from build123d import *
from OCP.BRepFilletAPI import BRepFilletAPI_MakeChamfer

# Parameters (mm, degrees)
BOSS_EXTRUDE1_DEPTH       = 33.86758938
F_1_4_CLEARANCE_HOLE1_D   = 7.14248
DRAFT1_ANGLE              = 15
DRAFT2_ANGLE              = 15
DRAFT3_ANGLE              = 5
DRAFT4_ANGLE              = 5
CHAMFER1_SIZE             = 2.54
CHAMFER1_SIZE2            = 2.599295174
CHAMFER2_SIZE             = 1.27
CHAMFER2_SIZE2            = 1.356155551
CHAMFER2_SIZE2_2          = 1.397079842
CHAMFER2_SIZE2_3          = 1.796051224
CHAMFER2_SIZE2_4          = 1.739452222
HOLE1_AT_2_COUNT          = 2
HOLE1_AT_2_PITCH          = 24.154432116
F_8_CLEARANCE_HOLE1_D     = 4.9149
F_8_CLEARANCE_HOLE1_DEPTH = 9.525
F_8_CLEARANCE_HOLE1_TIP   = 1.476584928


with BuildPart() as part:
    # Sketch1 → Boss-Extrude1 (new body)
    with BuildSketch(Plane.XY):
        Polygon((133.529465969, -12.7), (114.479465969, -12.7), (114.479465969, -8.89), (111.939465969, -6.35), (107.494465969, -6.35), (104.954465969, -6.35), (104.954465969, -25.4), (143.054465969, -25.4), (143.054465969, -6.35), (140.514465969, -6.35), (136.069465969, -6.35), (133.529465969, -8.89), align=None)
    extrude(amount=-BOSS_EXTRUDE1_DEPTH)

    # 1/4 Clearance Hole1 (through all)
    with Locations(Plane(origin=(0, -12.7, 0), x_dir=(1, 0, 0), z_dir=(0, 1, 0))):
        with Locations((124.004465969, 6.77379469), (124.004465969, 27.09379469)):
            Hole(F_1_4_CLEARANCE_HOLE1_D / 2)

    # Draft1
    draft1_faces = [part.faces().sort_by_distance(p)[0] for p in [
        (143.054465969, -15.875, -16.93379469),
    ]]
    draft(draft1_faces, Plane(origin=(140.514465969, -6.35, -76.464684351), x_dir=(1, 0, 0), z_dir=(0, 1, 0)), DRAFT1_ANGLE)

    # Draft2
    draft2_faces = [part.faces().sort_by_distance(p)[0] for p in [
        (104.954465969, -15.875, -16.93379469),
    ]]
    draft(draft2_faces, Plane(origin=(140.514465969, -6.35, -76.464684351), x_dir=(1, 0, 0), z_dir=(0, 1, 0)), DRAFT2_ANGLE)

    # Draft3
    draft3_faces = [part.faces().sort_by_distance(p)[0] for p in [
        (124.004465969, -17.503560526, 0),
    ]]
    draft(draft3_faces, Plane(origin=(140.514465969, -6.35, -76.464684351), x_dir=(1, 0, 0), z_dir=(0, 1, 0)), DRAFT3_ANGLE)

    # Draft4
    draft4_faces = [part.faces().sort_by_distance(p)[0] for p in [
        (124.004465969, -17.503560526, -33.86758938),
    ]]
    draft(draft4_faces, Plane(origin=(140.514465969, -6.35, -76.464684351), x_dir=(1, 0, 0), z_dir=(0, 1, 0)), DRAFT4_ANGLE)

    # Chamfer1: one chamfer whose edges measure the first distance from different faces: ONE call of the kernel's chamfer builder (chamfer() names one face for all edges)
    chamfer1_edges_1 = [part.edges().sort_by_distance(p)[0] for p in [
        (145.606682027, -15.875, 0.83332952),
        (145.606682027, -15.875, -34.7009189),
    ]]
    chamfer1_side_1 = [part.faces().sort_by_distance(p)[0] for p in [
        (145.646584132, -16.023916684, -16.93379469),
    ]]
    chamfer1_edges_2 = [part.edges().sort_by_distance(p)[0] for p in [
        (102.402249911, -15.875, 0.83332952),
        (102.402249911, -15.875, -34.7009189),
    ]]
    chamfer1_side_2 = [part.faces().sort_by_distance(p)[0] for p in [
        (102.362347806, -16.023916684, -16.93379469),
    ]]
    chamfer1 = BRepFilletAPI_MakeChamfer(part.part.solid().wrapped)
    for e in chamfer1_edges_1:
        chamfer1.Add(CHAMFER1_SIZE, CHAMFER1_SIZE2, e.wrapped, chamfer1_side_1[0].wrapped)  # the first distance lies on this face
    for e in chamfer1_edges_2:
        chamfer1.Add(CHAMFER1_SIZE, CHAMFER1_SIZE2, e.wrapped, chamfer1_side_2[0].wrapped)  # the first distance lies on this face
    add(Compound.cast(chamfer1.Shape()), mode=Mode.REPLACE)

    # Chamfer2: one chamfer whose edges measure the first distance from different faces: ONE call of the kernel's chamfer builder (chamfer() names one face for all edges)
    chamfer2_edges_1 = [part.edges().sort_by_distance(p)[0] for p in [
        (134.799465969, -7.62, 0.111110603),
        (134.799465969, -7.62, -33.978699983),
    ]]
    chamfer2_side_1 = [part.faces().sort_by_distance(p)[0] for p in [
        (134.796706387, -7.622759582, -16.93379469),
    ]]
    chamfer2_edges_2 = [part.edges().sort_by_distance(p)[0] for p in [
        (109.792117792, -6.35, 0),
        (109.792117792, -6.35, -33.86758938),
    ]]
    chamfer2_side_2 = [part.faces().sort_by_distance(p)[0] for p in [
        (108.524459453, -6.35, -16.93379469),
    ]]
    chamfer2_edges_3 = [part.edges().sort_by_distance(p)[0] for p in [
        (113.209465969, -7.62, 0.111110603),
        (113.209465969, -7.62, -33.978699983),
    ]]
    chamfer2_side_3 = [part.faces().sort_by_distance(p)[0] for p in [
        (113.212225552, -7.622759582, -16.93379469),
    ]]
    chamfer2_edges_4 = [part.edges().sort_by_distance(p)[0] for p in [
        (114.479465969, -10.795, 0.388887109),
        (133.529465969, -10.795, 0.388887109),
        (114.479465969, -10.795, -34.256476489),
        (133.529465969, -10.795, -34.256476489),
    ]]
    chamfer2_edges_5 = [part.edges().sort_by_distance(p)[0] for p in [
        (124.004465969, -12.7, 0.555553013),
        (124.004465969, -12.7, -34.423142393),
    ]]
    chamfer2_side_5 = [part.faces().sort_by_distance(p)[0] for p in [
        (124.004465969, -12.7, -16.93379469),
    ]]
    chamfer2_edges_6 = [part.edges().sort_by_distance(p)[0] for p in [
        (138.216814146, -6.35, -33.86758938),
        (138.216814146, -6.35, 0),
    ]]
    chamfer2_side_6 = [part.faces().sort_by_distance(p)[0] for p in [
        (139.484472486, -6.35, -16.93379469),
    ]]
    chamfer2_edges_7 = [part.edges().sort_by_distance(p)[0] for p in [
        (104.954465969, -6.35, -16.93379469),
    ]]
    chamfer2_side_7 = [part.faces().sort_by_distance(p)[0] for p in [
        (102.355664133, -16.048860491, -16.93379469),
    ]]
    chamfer2_edges_8 = [part.edges().sort_by_distance(p)[0] for p in [
        (106.299617792, -6.35, -1.274526802),
    ]]
    chamfer2_side_8 = [part.faces().sort_by_distance(p)[0] for p in [
        (103.747401735, -15.875, -0.441197282),
    ]]
    chamfer2_edges_9 = [part.edges().sort_by_distance(p)[0] for p in [
        (106.299617792, -6.35, -32.593062578),
    ]]
    chamfer2_side_9 = [part.faces().sort_by_distance(p)[0] for p in [
        (103.747401735, -15.875, -33.426392098),
    ]]
    chamfer2_edges_10 = [part.edges().sort_by_distance(p)[0] for p in [
        (143.054465969, -6.35, -16.93379469),
    ]]
    chamfer2_side_10 = [part.faces().sort_by_distance(p)[0] for p in [
        (139.484472486, -6.35, -16.93379469),
    ]]
    chamfer2_edges_11 = [part.edges().sort_by_distance(p)[0] for p in [
        (141.709314146, -6.35, -1.274526802),
    ]]
    chamfer2_side_11 = [part.faces().sort_by_distance(p)[0] for p in [
        (144.261530204, -15.875, -0.441197282),
    ]]
    chamfer2_edges_12 = [part.edges().sort_by_distance(p)[0] for p in [
        (141.709314146, -6.35, -32.593062578),
    ]]
    chamfer2_side_12 = [part.faces().sort_by_distance(p)[0] for p in [
        (144.261530204, -15.875, -33.426392098),
    ]]
    chamfer2 = BRepFilletAPI_MakeChamfer(part.part.solid().wrapped)
    for e in chamfer2_edges_1:
        chamfer2.Add(CHAMFER2_SIZE, CHAMFER2_SIZE2, e.wrapped, chamfer2_side_1[0].wrapped)  # the first distance lies on this face
    for e in chamfer2_edges_2:
        chamfer2.Add(CHAMFER2_SIZE, CHAMFER2_SIZE2_2, e.wrapped, chamfer2_side_2[0].wrapped)  # the first distance lies on this face
    for e in chamfer2_edges_3:
        chamfer2.Add(CHAMFER2_SIZE, CHAMFER2_SIZE2, e.wrapped, chamfer2_side_3[0].wrapped)  # the first distance lies on this face
    for e in chamfer2_edges_4:
        chamfer2.Add(CHAMFER2_SIZE, e.wrapped)
    for e in chamfer2_edges_5:
        chamfer2.Add(CHAMFER2_SIZE, CHAMFER2_SIZE2_2, e.wrapped, chamfer2_side_5[0].wrapped)  # the first distance lies on this face
    for e in chamfer2_edges_6:
        chamfer2.Add(CHAMFER2_SIZE, CHAMFER2_SIZE2_2, e.wrapped, chamfer2_side_6[0].wrapped)  # the first distance lies on this face
    for e in chamfer2_edges_7:
        chamfer2.Add(CHAMFER2_SIZE, CHAMFER2_SIZE2_3, e.wrapped, chamfer2_side_7[0].wrapped)  # the first distance lies on this face
    for e in chamfer2_edges_8:
        chamfer2.Add(CHAMFER2_SIZE, CHAMFER2_SIZE2_4, e.wrapped, chamfer2_side_8[0].wrapped)  # the first distance lies on this face
    for e in chamfer2_edges_9:
        chamfer2.Add(CHAMFER2_SIZE, CHAMFER2_SIZE2_4, e.wrapped, chamfer2_side_9[0].wrapped)  # the first distance lies on this face
    for e in chamfer2_edges_10:
        chamfer2.Add(CHAMFER2_SIZE, CHAMFER2_SIZE2_3, e.wrapped, chamfer2_side_10[0].wrapped)  # the first distance lies on this face
    for e in chamfer2_edges_11:
        chamfer2.Add(CHAMFER2_SIZE, CHAMFER2_SIZE2_4, e.wrapped, chamfer2_side_11[0].wrapped)  # the first distance lies on this face
    for e in chamfer2_edges_12:
        chamfer2.Add(CHAMFER2_SIZE, CHAMFER2_SIZE2_4, e.wrapped, chamfer2_side_12[0].wrapped)  # the first distance lies on this face
    add(Compound.cast(chamfer2.Shape()), mode=Mode.REPLACE)

    # Sketch5 → Hole1 (revolve, cut)
    with BuildSketch(Plane(origin=(111.927249911, -25.4, -16.93379469), x_dir=(0, 0, -1), z_dir=(1, 0, 0))):
        Polygon((0, 0), (0, 4.699), (2.8702, 4.699), (2.9972, 0), align=None)
    hole1 = revolve(axis=Axis((111.927249911, 84.6, -16.93379469), (0, -1, 0)), mode=Mode.SUBTRACT)

    # Hole1 at 2: Hole1 ×2
    with Locations(*[(i * HOLE1_AT_2_PITCH, 0, 0) for i in range(1, HOLE1_AT_2_COUNT)]):
        add(hole1, mode=Mode.SUBTRACT)

    # #8 Clearance Hole1
    with Locations(Plane(origin=(0, -25.4, 0), x_dir=(-1, 0, 0), z_dir=(0, -1, 0))):
        with Locations((-136.081682027, 16.93379469), (-111.927249911, 16.93379469)):
            Hole(F_8_CLEARANCE_HOLE1_D / 2, depth=F_8_CLEARANCE_HOLE1_DEPTH)
            with Locations((0, 0, -(F_8_CLEARANCE_HOLE1_DEPTH + F_8_CLEARANCE_HOLE1_TIP / 2))):  # 118° drill point
                Cone(0, F_8_CLEARANCE_HOLE1_D / 2, F_8_CLEARANCE_HOLE1_TIP, mode=Mode.SUBTRACT)


solid = part.part
Can you work these out from the model? Positions are in its coordinate system, mm. A direction names the side the tool comes from. Round coordinates to 2 decimals unless told otherwise and drop trailing zeros. Write each loop counter-clockwise with the first axis right and the second up, starting at its lowest first coordinate (ties: lowest second). Pieces come first, ordered by that corner, then holes. Notation, with made-up numbers: (-19.5, 16) -> (22.5, 16) arc R24 ccw to (22.5, 42) -> close; hole circle Ø8 at (22, -35). An arc over 180 degrees is marked (long way). One line per question, with ' | ' between items. Start each with the question number.
1) I'm going to push flat-ended pins straight in: P1, Ø1.5, axis at y = -16.5, z = -26.5, coming from the -X side; P2, Ø1.9, axis at y = -10, z = -9, coming from the -X side; P3, Ø10, axis at y = -19, z = -8, coming from the +X side; P4, Ø3, axis at x = 110.5, z = -17.5, coming from the -Y side. Where does each tip first touch, or does it pass through?
2) On a 3-axis mill with a long thin cutter (end or side, diameter ignored), from which of +Z, -Z, +X, -X, +Y, -Y can I reach the whole of each face in a straight line? I mean faces 5 (the flat face through (134.156, -11.453, -0.2)), 6 (the flat face through (135.3, -8.1, -33.4)), 7 (the cylindrical face through (133.627, -18.254, -17.042)). Say none if no direction works.
3) If we mould it in two halves opening along Z, with no side actions, what happens to faces 1 (the flat face through (135.33, -8.06, -0.48)), 2 (the conical face through (111.52, -14.655, -17.062)), 3 (the flat face through (124, -25.4, -17)), 4 (the cylindrical face through (127.572, -19.139, -27.251))? For each: released by +Z, released by -Z, zero draft, split by the parting line, or undercut.
4) I need wall thicknesses on line 1 (Z direction, x = 123.5, y = -19.5); line 2 (Z direction, x = 122.5, y = -17.75); line 3 (Z direction, x = 110.5, y = -17.5). Which ranges of each line are inside material? Lowest first, please. Write a range as [from, to].
5) Suppose I cut it at B-B on z = -25.5. Write out the boundary of the cut face in (x, y), then the cut area to 3 significant figures.
6) Suppose I cut it at C-C on y = -19.25. Write out the boundary of the cut face in (x, z), then the cut area to 3 significant figures.
7) Suppose I cut it at A-A on y = -10.5. Write out the boundary of the cut face in (x, z).
8) Suppose I cut it at D-D on y = -22. Write out the boundary of the cut face in (x, z).
Return value:
1) P1: stops at x = 102.03 | P2: stops at x = 103.72 | P3: stops at x = 147.78 | P4: stops at y = -25.4
2) face 5: +Z, +Y | face 6: -Z, +Y | face 7: -Y
3) face 1: released by +Z | face 2: undercut | face 3: zero draft | face 4: undercut
4) line 1: z = [-35.02, -30.63], [-23.56, -10.31], [-3.24, 1.15] | line 2: z = [-34.86, -30.33], [-23.85, -10.01], [-3.53, 1] | line 3: z = [-34.84, -18.93], [-14.93, 0.98]
5) outline: (99.85, -25.4) -> (120.81, -25.4) -> (120.81, -12.7) -> (114.48, -12.7) -> (114.48, -8.89) -> (111.94, -6.35) -> (106.75, -6.35) -> (104.63, -7.58) -> close; (127.2, -25.4) -> (148.16, -25.4) -> (143.52, -8.08) -> (141.78, -6.35) -> (136.07, -6.35) -> (133.53, -8.89) -> (133.53, -12.7) -> (127.2, -12.7) -> close | area: 612 mm2
6) outline: (101.5, -32.45) -> (104.19, -35) -> (143.82, -35) -> (146.51, -32.45) -> (146.51, -1.42) -> (143.82, 1.13) -> (104.19, 1.13) -> (101.5, -1.42) -> close; hole circle Ø4.91 at (111.93, -16.93); hole circle Ø7.14 at (124, -27.09); hole circle Ø7.14 at (124, -6.77); hole circle Ø4.91 at (136.08, -16.93) | area: 1,490 mm2
7) outline: (103.84, -31.68) -> (106.53, -34.23) -> (113.21, -34.23) -> (114.48, -32.96) -> (114.48, -0.91) -> (113.21, 0.36) -> (106.53, 0.36) -> (103.84, -2.19) -> close; (133.53, -32.96) -> (134.8, -34.23) -> (141.48, -34.23) -> (144.17, -31.68) -> (144.17, -2.19) -> (141.48, 0.36) -> (134.8, 0.36) -> (133.53, -0.91) -> close
8) outline: (100.76, -32.69) -> (103.45, -35.24) -> (144.56, -35.24) -> (147.25, -32.69) -> (147.25, -1.18) -> (144.56, 1.37) -> (103.45, 1.37) -> (100.76, -1.18) -> close; hole circle Ø5.81 at (111.93, -16.93); hole circle Ø7.14 at (124, -27.09); hole circle Ø7.14 at (124, -6.77); hole circle Ø5.81 at (136.08, -16.93)
